Check sheet for the modelled part. Datum: model origin and axes. Units: mm. Face numbers are marked on the shaded views. A direction names the side the tool comes from. Round coordinates to 2 decimals unless told otherwise and drop trailing zeros. Loops run counter-clockwise (first coordinate to the right, second up) from the corner with the lowest first, then second, coordinate; pieces in that order, holes last. Notation, with made-up numbers: (23, -28.75) - (56, -28.75) arc R23 ccw to (56, -1.75) - close; hole circle Ø4 at (-39, 21). An arc over 180 degrees is marked (long way). Answer in a Markdown table with one row per item. Add a question column.
(1) Cross-section at A-A on x = -2.5. Enter the section's corners in (y, z).
(2) Cross-section at D-D on z = -1. Enter the section's corners in (x, y), then the cut area to 3 significant figures.
(3) Cross-section at C-C on x = 32. Enter the section's corners in (y, z).
(4) Access from +Z, -Z, +X, -X, +Y, -Y to the whole of each face (thin tool, end or side, straight path). Record for the marked faces 1, 2, 3 and 4.
(5) Cross-section at B-B on z = 12. Enter the section's corners in (x, y), then the cut area to 3 significant figures.
(6) Thickness scan on line 1 along Y through (x, z) = (32, 12); line 2 along Y through (x, z) = (-2.5, 9.15); line 3 along Y through (x, z) = (25, 4). Record the ranges inside material, lowest first.
(7) Gauge pin test, flat ends, axial feed: pin 1 (4 mm diameter, centred on x = 57, y = 2.5, fed in from +Z); pin 2 (1.8 mm diameter, centred on x = -2.5, y = 11.09, fed in from -Z); pin 3 (4 mm diameter, centred on x = 32, y = 8, fed in from -Z); pin 4 (4 mm diameter, centred on x = -2.5, y = 11, fed in from -Z). Record the tip position at first contact, or that the pin passes through.
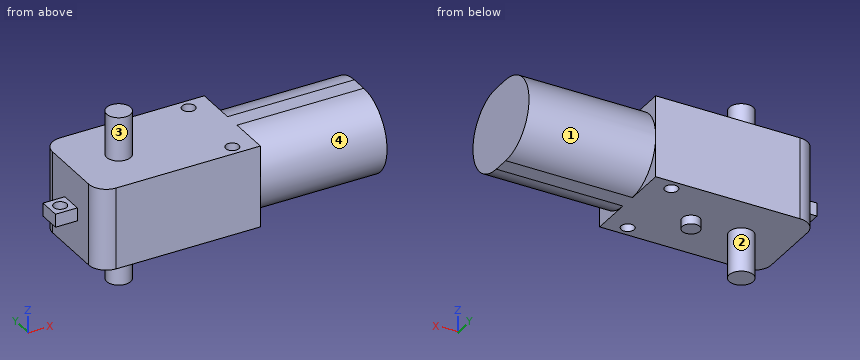
Autodesk Inventor part; units mm, degrees
ref_plane "YZ Plane" through (0, 0, 0) normal (1, 0, 0) x (0, 1, 0)
ref_plane "XZ Plane" through (0, 0, 0) normal (0, 1, 0) x (-1, 0, 0)
ref_plane "XY Plane" through (0, 0, 0) normal (0, 0, 1) x (1, 0, 0)
sketch "Skizze1" plane through (0, 0, 0) normal (0, 0, 1) x (1, 0, 0)
  line L0 (0, 0) -> (37, 0)
  line L1 (37, 0) -> (37, 22.5)
  line L2 (37, 22.5) -> (0, 22.5)
  line L3 (0, 22.5) -> (0, 0)
  dimension "d0" = 37
  dimension "d1" = 22.5
extrude "Extrusion1" add sketch "Skizze1" along normal blind 18.7
sketch "Skizze2" plane through (37, 0, 0) normal (1, 0, 0) x (0, 0, -1)
  line L0 (0, 0) -> (0, 22.5)
  line L1 (-9.35, 13.157) -> (-9.35, 9.3514) construction
  line L2 (-18.7, 13.157) -> (-18.7, 9.3514)
  line L3 (0, 9.3514) -> (0, 13.157)
  arc A0 (0, 13.157) -> (-18.7, 13.157) centre (-9.35, 13.157) ccw
  arc A1 (-18.7, 9.3514) -> (0, 9.3514) centre (-9.35, 9.3514) ccw
  point P0 (-9.35, 11.2542)
extrude "Extrusion2" add sketch "Skizze2" along normal blind 29
sketch "Skizze3" plane through (0, 0, 18.7) normal (0, 0, 1) x (1, 0, 0)
  line L0 (37, 22.5) -> (0, 22.5)
  line L1 (0, 22.5) -> (0, 0)
  circle A0 centre (11, 11.25) radius 2.75
  dimension "d6" = 11
  dimension "d7" = 11.25
  dimension "d21" = 5.5
extrude "Extrusion3" add sketch "Skizze3" along normal blind 10
sketch "Skizze4" plane through (0, 0, 0) normal (0, 0, -1) x (-1, 0, 0)
  line L0 (0, 0) -> (-37, 0)
  line L1 (0, 22.5) -> (0, 0)
  circle A0 centre (-11, 11.25) radius 2.75
  dimension "d10" = 5.5
  dimension "d11" = 11
  dimension "d12" = 11.25
extrude "Extrusion4" add sketch "Skizze4" along normal blind 10
sketch "Skizze5" plane through (0, 0, 0) normal (0, 0, -1) x (-1, 0, 0)
  line L0 (0, 0) -> (-37, 0)
  line L1 (0, 22.5) -> (0, 0)
  line L2 (-37, 22.5) -> (0, 22.5)
  circle A0 centre (-22.5, 11.25) radius 2
  dimension "d15" = 4
  dimension "d16" = 11.25
  dimension "d17" = 22.5
  dimension "d18" = 11.25
extrude "Extrusion5" add sketch "Skizze5" along normal blind 2
sketch "Skizze6" plane through (0, 0, 0) normal (-1, 0, 0) x (0, 0, 1)
  line L0 (0, 22.5) -> (0, 0)
  line L1 (18.7, 22.5) -> (18.7, 0)
  line L2 (7.85, 13.5868) -> (10.85, 13.5868)
  line L3 (10.85, 13.5868) -> (10.85, 8.5868)
  line L4 (10.85, 8.5868) -> (7.85, 8.5868)
  line L5 (7.85, 8.5868) -> (7.85, 13.5868)
  line L6 (9.35, 13.5868) -> (9.35, 8.5868)
  dimension "d22" = 3
  dimension "d23" = 5
  dimension "d25" = 18.7
  dimension "d26" = 7.85
  dimension "d27" = 7.85
extrude "Extrusion6" add sketch "Skizze6" along normal blind 5
fillet "Rundung1" radius 4 2 edges at (0, 22.5, 9.35) (0, 0, 9.35)
sketch "Skizze7" plane through (0, 0, 18.7) normal (0, 0, 1) x (1, 0, 0)
  line L0 (4, 0) -> (37, 0)
  line L1 (37, 22.5) -> (4, 22.5)
  line L2 (0, 18.5) -> (0, 4)
  circle A0 centre (32, 20) radius 1.5
  circle A1 centre (32, 2.5) radius 1.5
  point P0 (0, 0)
  dimension "d31" = 2.5
  dimension "d32" = 2.5
  dimension "d33" = 32
  dimension "d34" = 32
  dimension "d35" = 3
  dimension "d36" = 3
extrude "Extrusion7" cut sketch "Skizze7" against normal up to next
hole "Bohrung1" at (-2.5, 11.0868, 10.85) direction (0, 0, -1) diameter 3 end through all
properties part number "Motor_gerade"
Answers:
| question | item | result |
|---|---|---|
| 1 | outline | (8.59, 7.85) - (9.59, 7.85) - (9.59, 10.85) - (8.59, 10.85) - close; (12.59, 7.85) - (13.59, 7.85) - (13.59, 10.85) - (12.59, 10.85) - close |
| 2 | outline | circle Ø5.5 at (11, 11.25); circle Ø4 at (22.5, 11.25) |
| 2 | area | 36.3 mm^2 |
| 3 | outline | (0, 0) - (1, 0) - (1, 18.7) - (0, 18.7) - close; (4, 0) - (18.5, 0) - (18.5, 18.7) - (4, 18.7) - close; (21.5, 0) - (22.5, 0) - (22.5, 18.7) - (21.5, 18.7) - close |
| 4 | face 1 | +X, +Y |
| 4 | face 2 | -Z |
| 4 | face 3 | +Z |
| 4 | face 4 | +X, -Y |
| 5 | outline | (0, 4) arc R4 ccw to (4, 0) - (37, 0) - (37, 0.38) - (66, 0.38) - (66, 22.12) - (37, 22.12) - (37, 22.5) - (4, 22.5) arc R4 ccw to (0, 18.5) - close; hole circle Ø3 at (32, 2.5); hole circle Ø3 at (32, 20) |
| 5 | area | 1,440 mm^2 |
| 6 | line 1 | y = 0 to 1, 4 to 18.5, 21.5 to 22.5 |
| 6 | line 2 | y = 8.59 to 9.59, 12.59 to 13.59 |
| 6 | line 3 | y = 0 to 22.5 |
| 7 | pin 1 | stops at z = 17.34 |
| 7 | pin 2 | passes through |
| 7 | pin 3 | stops at z = 0 |
| 7 | pin 4 | stops at z = 7.85 |
